from build123d import *

# Parameters (mm, degrees)
F0_R     = 50.8
F1_DEPTH = 38.1
F2_W     = 63.5
F2_H     = 76.2
F3_DEPTH = 203.2
F4_R     = 38.1
F5_DEPTH = 19.05
F6_R     = 38.1
F7_DEPTH = 19.05


with BuildPart() as f1:
    # F0 (on Right) → F1 (new body, symmetric)
    with BuildSketch(Plane.YZ):
        Circle(F0_R)
    extrude(amount=F1_DEPTH, both=True)

    # F2 (on Top) → F3 (join)
    with BuildSketch(Plane.XY):
        Rectangle(F2_W, F2_H)
    extrude(amount=-F3_DEPTH)

    # F4 (on face) → F5 (join)
    with BuildSketch(Plane(origin=(-31.75, 0, 0), x_dir=(0, -1, 0), z_dir=(-1, 0, 0))):
        with Locations((0, -203.2)):
            Circle(F4_R)
    extrude(amount=-F5_DEPTH)

    # F6 (on face) → F7 (join)
    with BuildSketch(Plane.YZ.offset(31.75)):
        with Locations((0, -203.2)):
            Circle(F6_R)
    extrude(amount=-F7_DEPTH)


solid = f1.part
The listing builds one solid part. Answer for the finished solid, in the listing's coordinates (mm). A direction names the side the tool comes from. Coordinates: 2 decimals unless noted, no trailing zeros. Loops run counter-clockwise (first coordinate to the right, second up) from the corner with the lowest first, then second, coordinate; pieces in that order, holes last.
1) Find section D-D on y = -12.5. Write down the section's boundary in (x, z), then the cut area to 3 significant figures.
2) Determine the mould class of faces 1 (the face through (12.7, -1, -218)), 2 (the face through (31.75, -1, -136)), 3 (the face through (22.36, -0.84, -241.29)) for opening direction X: pulls with the +X half, pulls with the -X half, needs draft (parallel to the pull), parting line crosses it, or undercut.
3) Find section C-C on z = -58.5. Write down the section's boundary in (x, y), then the cut area to 3 significant figures.
4) A tool of negligible diameter and unlimited length cuts with its end or side. For faces 4 (the face through (0, -38.1, -117)), 5 (the face through (-22.36, 0.84, -241.29)), 6 (the face through (0, 1, -203.2)), 7 (the face through (0, 38.1, -117)), from which of +Z, -Z, +X, -X, +Y, -Y can it reach the whole face along a straight path? Write none if from no direction.
5) Find the intervals of material crossed by L1, parallel to X at y = 23, z = -218; L2, parallel to X at y = 3, z = -84; L3, parallel to Y at x = 21, z = -85, in increasing order.
6) Find section A-A on y = 0. Write down the section's boundary in (x, z), then the cut area to 3 significant figures.
7) Flat-ended cylindrical pins translate along their axes: pin 1 Ø11.5 at (y, z) = (17, -227.5) entering from +X; pin 2 Ø11.5 at (y, z) = (15.5, -219.5) entering from -X; pin 3 Ø8 at (x, y) = (22, 2.5) entering from +Z. Find the tip coordinate at first contact, or state that the pin passes through.
8) Find section B-B on x = -9. Write down the section's boundary in (y, z).
Values:
1. outline: (-38.1, -49.24) - (-31.75, -49.24) - (-31.75, -239.19) - (-12.7, -239.19) - (-12.7, -203.2) - (12.7, -203.2) - (12.7, -239.19) - (31.75, -239.19) - (31.75, -49.24) - (38.1, -49.24) - (38.1, 49.24) - (-38.1, 49.24) - close
1. area: 18,700 mm2
2. face 1: undercut
2. face 2: pulls with the +X half
2. face 3: needs draft
3. outline: (-31.75, -38.1) - (31.75, -38.1) - (31.75, 38.1) - (-31.75, 38.1) - close
3. area: 4,840 mm2
4. face 4: -Z, +X, -X, -Y
4. face 5: -Z, +X, -X
4. face 6: -Z, +Y, -Y
4. face 7: -Z, +X, -X, +Y
5. L1: x = -31.75 to -12.7, 12.7 to 31.75
5. L2: x = -31.75 to 31.75
5. L3: y = -38.1 to 38.1
6. outline: (-38.1, -50.8) - (-31.75, -50.8) - (-31.75, -241.3) - (-12.7, -241.3) - (-12.7, -203.2) - (12.7, -203.2) - (12.7, -241.3) - (31.75, -241.3) - (31.75, -50.8) - (38.1, -50.8) - (38.1, 50.8) - (-38.1, 50.8) - close
6. area: 18,900 mm2
7. pin 1: stops at x = 31.75
7. pin 2: stops at x = -31.75
7. pin 3: stops at z = 50.8
8. outline: (-38.1, -203.2) - (38.1, -203.2) - (38.1, -33.6) arc R50.8 ccw (long way) to (-38.1, -33.6) - close
